Geometry: final body of the model. Coordinates: model frame, mm. Face numbers are marked on the shaded views. A direction names the side the tool comes from. Give positions to 0.01 mm unless a question says otherwise; leave off trailing zeros. Write each loop counter-clockwise with the first axis right and the second up, starting at its lowest first coordinate (ties: lowest second). Pieces come first, ordered by that corner, then holes.
Q1. Cut plane B-B on x = 25. Return the cut outline in (y, z).
Q2. Pin query (flat end, axial travel): pin 1 (2 mm diameter, centred on x = 38.5, z = 44.5, fed in from +Y). Return the tip coordinate at first contact, or that it passes through.
Q3. Cut plane C-C on y = 20. Return the cut outline in (x, z).
Q4. Cut plane A-A on z = 25. Return the cut outline in (x, y).
Q5. Reachability of the marked faces 5 and 6 from +Z, -Z, +X, -X, +Y, -Y: full face, straight path, thin tool, end or side. Return the list, or none.
Q6. Draft query along Y for the marked faces 1, 2, 3 and 4. Return one class per face: pulls with the +Y half, pulls with the -Y half, needs draft (parallel to the pull), parting line crosses it, or undercut.
Q7. Cut plane D-D on z = 11.5. Return the cut outline in (x, y).
Q8. Line query: L1, parallel to X at y = -7, z = 25; L2, parallel to Y at x = -6, z = 25; L3, parallel to X at y = 60.5, z = 46.5. Output: solid intervals per line, ascending.
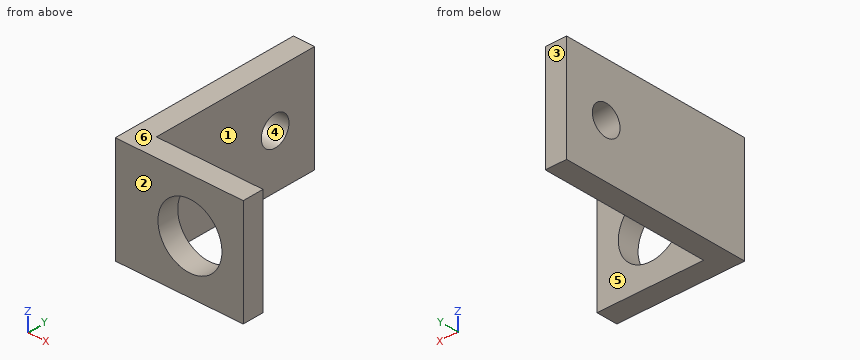
```python
from build123d import *

# Parameters (mm, degrees)
EXTRUDE_THIN1_DEPTH = 50
SKETCH2_R           = 15
CUT_EXTRUDE1_DEPTH  = 107.77078252
SKETCH3_R           = 7
CUT_EXTRUDE2_DEPTH  = 107.77078252


with BuildPart() as part:
    # Sketch1 → Extrude-Thin1 (new body)
    with BuildSketch(Plane.XY):
        Polygon((0, 80), (0, 0), (50, 0), (50, -10), (-10, -10), (-10, 80), align=None)
    extrude(amount=EXTRUDE_THIN1_DEPTH)

    # Sketch2 → Cut-Extrude1 (cut, through all)
    with BuildSketch(Plane(origin=(0, 0, 0), x_dir=(1, 0, 0), z_dir=(0, 1, 0))):
        with Locations(Location((25, -25, 0), (0, 0, 270))):
            Circle(SKETCH2_R)
    extrude(amount=-CUT_EXTRUDE1_DEPTH, mode=Mode.SUBTRACT)

    # Sketch3 → Cut-Extrude2 (cut, through all)
    with BuildSketch(Plane(origin=(0, 0, 0), x_dir=(0, 0, -1), z_dir=(1, 0, 0))):
        with Locations((-25, 60)):
            Circle(SKETCH3_R)
    extrude(amount=-CUT_EXTRUDE2_DEPTH, mode=Mode.SUBTRACT)


solid = part.part
```
Data:
1. outline: (-10, 0) - (0, 0) - (0, 10) - (-10, 10) - close; (-10, 40) - (0, 40) - (0, 50) - (-10, 50) - close
2. pin 1: stops at y = 0
3. outline: (-10, 0) - (0, 0) - (0, 50) - (-10, 50) - close
4. outline: (-10, -10) - (10, -10) - (10, 0) - (0, 0) - (0, 53) - (-10, 53) - close; (-10, 67) - (0, 67) - (0, 80) - (-10, 80) - close; (40, -10) - (50, -10) - (50, 0) - (40, 0) - close
5. face 5: +Z, -Z, +X, +Y
5. face 6: +Z, +X, -X, +Y, -Y
6. face 1: needs draft
6. face 2: pulls with the -Y half
6. face 3: pulls with the +Y half
6. face 4: undercut
7. outline: (-10, -10) - (18.46, -10) - (18.46, 0) - (0, 0) - (0, 80) - (-10, 80) - close; (31.54, -10) - (50, -10) - (50, 0) - (31.54, 0) - close
8. L1: x = -10 to 10, 40 to 50
8. L2: y = -10 to 53, 67 to 80
8. L3: x = -10 to 0
